from build123d import *

# Parameters (mm, degrees)
F0_R     = 3
F1_DEPTH = 5
F2_R     = 2
F3_DEPTH = 5
F4_SIZE  = 0.5
F5_SIZE  = 0.2


with BuildPart() as f1:
    # F0 (on Top) → F1 (new body)
    with BuildSketch(Plane.XY):
        Circle(F0_R)
    extrude(amount=F1_DEPTH)

    # F2 (on Top) → F3 (join)
    with BuildSketch(Plane.XY):
        Circle(F2_R)
    extrude(amount=-F3_DEPTH)

    # F4
    f4_edges = [f1.edges().sort_by_distance(p)[0] for p in [
        (-3, 0, 5),
    ]]
    chamfer(f4_edges, length=F4_SIZE)

    # F5
    f5_edges = [f1.edges().sort_by_distance(p)[0] for p in [
        (-2, 0, -5),
    ]]
    chamfer(f5_edges, length=F5_SIZE)


solid = f1.part
Verification items for the finished model (mm, model axes). A direction names the side the tool comes from. Give positions to 0.01 mm unless a question says otherwise; leave off trailing zeros. Loops run counter-clockwise (first coordinate to the right, second up) from the corner with the lowest first, then second, coordinate; pieces in that order, holes last.
1. Go/stop test with a flat-tipped pin: P1, Ø3, axis at y = -2.5, z = -1, coming from the -X side. Record where the tip stops, or that it passes through.
Derived:
P1: stops at x = -2.66
2. Cross-section at C-C on z = -3.5. Record the cut outline in (x, y), and give its area (3 significant figures).
Derived:
outline: circle Ø4 at (0, 0)
area: 12.6 mm2
3. Tool access check on faces 1 (the flat face through (1, -2, 0)), 2 (the flat face through (0, 0, -5)). Record the directions out of +Z, -Z, +X, -X, +Y, -Y that give a thin tool (end or side, any length) a straight path to the whole face; none if there is none.
Derived:
face 1: -Z
face 2: -Z, +X, -X, +Y, -Y
4. Cross-section at D-D on z = 3. Record the cut outline in (x, y).
Derived:
outline: circle Ø6 at (0, 0)
5. Material ranges on probe 1 along Z at (x, y) = (0.25, -2.35); probe 2 along Y at (x, z) = (0.1, -0.25); probe 3 along Y at (x, z) = (1.8, -3), recorded low to high.
Derived:
probe 1: z = 0 to 5
probe 2: y = -2 to 2
probe 3: y = -0.87 to 0.87
6. Cross-section at A-A on y = 0. Record the cut outline in (x, z), and give its area (3 significant figures).
Derived:
outline: (-3, 0) - (-2, 0) - (-2, -4.8) - (-1.8, -5) - (1.8, -5) - (2, -4.8) - (2, 0) - (3, 0) - (3, 4.5) - (2.5, 5) - (-2.5, 5) - (-3, 4.5) - close
area: 49.7 mm2
